from build123d import *

# Parameters (mm, degrees)
CHAMFER_1_SIZE = 1
CHAMFER_2_SIZE = 1


with BuildPart() as part:
    # 草图1 → 旋转1 (revolve)
    with BuildSketch(Plane.XY):
        Polygon((0, 0), (-4, 0), (-4, 13), (-6, 13), (-6, 14.5), (-3, 14.5), (-3, 50), (0, 50), align=None)
    revolve(axis=Axis((0, 50, 0), (0, -1, 0)))

    # 倒角1
    chamfer_1_edges = [part.edges().sort_by_distance(p)[0] for p in [
        (4, 0, 0),
    ]]
    chamfer(chamfer_1_edges, length=CHAMFER_1_SIZE)

    # 倒角2
    chamfer_2_edges = [part.edges().sort_by_distance(p)[0] for p in [
        (3, 50, 0),
    ]]
    chamfer(chamfer_2_edges, length=CHAMFER_2_SIZE)


solid = part.part
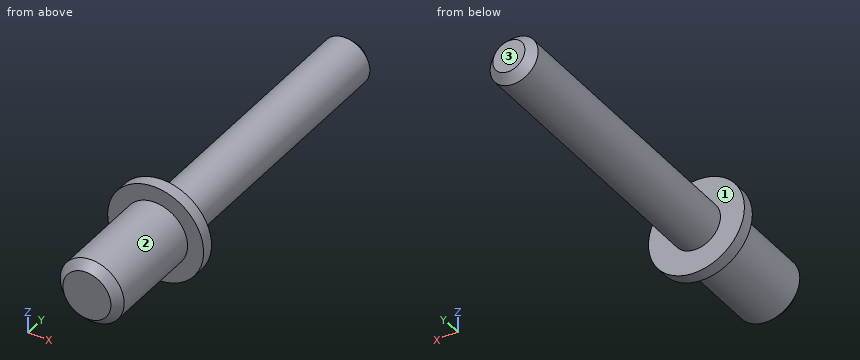
Model file for the job. Use its own axes, mm. Face numbers are marked on the shaded views. A direction names the side the tool comes from. Coordinates: 2 decimals unless noted, no trailing zeros. Write each loop counter-clockwise with the first axis right and the second up, starting at its lowest first coordinate (ties: lowest second). Pieces come first, ordered by that corner, then holes. Notation, with made-up numbers: (18, 39) -> (48, 39) arc R12 cw to (48, 62) -> close; hole circle Ø6 at (-22.75, 22). An arc over 180 degrees is marked (long way). One line per item, written item: value. Start each with the question number.
1) Flat gauge pins, fed straight in: pin 1 Ø6 at (x, y) = (-0.5, 12.5) entering from -Z; pin 2 Ø3 at (y, z) = (11, -4) entering from +X; pin 3 Ø1 at (y, z) = (40.5, 1.5) entering from +X; pin 4 Ø4 at (x, z) = (4.5, -3) entering from -Y. Where does each tip first touch, or does it go through?
2) Probe probe 1 along X at (y, z) = (22.5, 0.25); probe 2 along Y at (x, z) = (0.5, 4.5). List the from-to ranges inside material, lowest first.
3) Slice it at A-A on z = 0. Write the cut outline in (x, y).
4) Slice it at C-C on y = 6. Write the cut outline in (x, z), then the cut area to 3 significant figures.
5) Slice it at B-B on x = 0. Write the cut outline in (y, z), then the cut area to 3 significant figures.
6) Slice it at D-D on y = 38.5. Write the cut outline in (x, z).
7) Which spindle directions (+Z, -Z, +X, -X, +Y, -Y) get a long thin tool onto all of the face, cutting with end or side? Do the marked faces 1, 2 and 3. Say none if no direction does.
Answers follow:
1. pin 1: z = -6
1. pin 2: x = 3.12
1. pin 3: x = 2.83
1. pin 4: y = 0.41
2. probe 1: -2.99 to 2.99
2. probe 2: 13 to 14.5
3. outline: (-6, 13) -> (-4, 13) -> (-4, 1) -> (-3, 0) -> (3, 0) -> (4, 1) -> (4, 13) -> (6, 13) -> (6, 14.5) -> (3, 14.5) -> (3, 49) -> (2, 50) -> (-2, 50) -> (-3, 49) -> (-3, 14.5) -> (-6, 14.5) -> close
4. outline: circle Ø8 at (0, 0)
4. area: 50.3 mm2
5. outline: (0, -3) -> (1, -4) -> (13, -4) -> (13, -6) -> (14.5, -6) -> (14.5, -3) -> (49, -3) -> (50, -2) -> (50, 2) -> (49, 3) -> (14.5, 3) -> (14.5, 6) -> (13, 6) -> (13, 4) -> (1, 4) -> (0, 3) -> close
5. area: 333 mm2
6. outline: circle Ø6 at (0, 0)
7. face 1: +Y
7. face 2: -Y
7. face 3: +Z, -Z, +X, -X, +Y
